For this review, take the finished solid that the model builds, in its own axes (mm). Face numbers are marked on the shaded views. A direction names the side the tool comes from. Round coordinates to 2 decimals unless told otherwise and drop trailing zeros. Order: outer loops, then holes, each group sorted by start corner. A loop starts at its lowest first (then second) coordinate and runs counter-clockwise, first axis right, second up. Notation, with made-up numbers: (10.5, 40) -> (42.5, 40) arc R28 ccw to (42.5, 64) -> close; hole circle Ø8 at (-17.75, 25). An arc over 180 degrees is marked (long way). Answer in a Markdown table with one row per item.
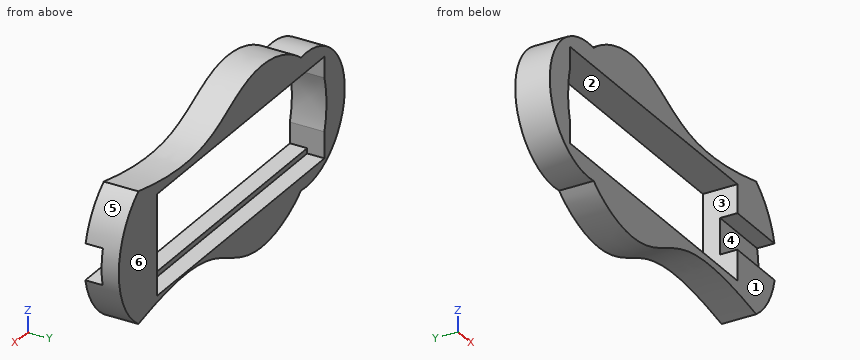
```python
from build123d import *

# Parameters (mm, degrees)
BOSS_EXTRUDE1_DEPTH = 20
SKETCH4_W           = 165
SKETCH4_H           = 3
CUT_EXTRUDE1_DEPTH  = 10
SKETCH9_W           = 41.41609898
SKETCH9_H           = 20.816936128
CUT_EXTRUDE2_DEPTH  = 10


with BuildPart() as part:
    # Sketch1 → Boss-Extrude1 (new body)
    with BuildSketch(Plane(origin=(0, 0, 0), x_dir=(1, 0, 0), z_dir=(0, 1, 0))):
        with BuildLine():
            add(Edge.make_bspline(
                [(145.295936906, 60.832177948), (44.156138469, 37.635123873), (68.598543861, 81.474917307), (14.861380224, 85.461006577), (-14.944677718, 60.924621218)],
                knots=[0, 0, 0, 0, 0, 1, 1, 1, 1, 1], degree=4))
            ThreePointArc((-14.944677718, 60.924621218), (-58.213287959, 23.039876711), (-14.944677718, -14.844867796))
            add(Edge.make_bspline(
                [(145.295936906, -14.752424526), (44.156138469, 8.444629549), (68.598543861, -35.395163885), (14.861380224, -39.381253155), (-14.944677718, -14.844867796)],
                knots=[0, 0, 0, 0, 0, 1, 1, 1, 1, 1], degree=4))
            ThreePointArc((145.295936906, -14.752424526), (164.569452441, 23.039876711), (145.295936906, 60.832177948))
        make_face()
        with BuildLine():
            Line((-38.21027036, -4.460123289), (-38.21027036, 7.689608728))
            add(Edge.make_bspline(
                [(-38.21027036, 38.390144694), (-42.352238314, 23.039876711), (-38.21027036, 7.689608728)],
                knots=[4.204471846, 4.204471846, 4.204471846, 5.220306115, 5.220306115, 5.220306115], degree=2, weights=[1, 0.873759421, 1]))
            Line((-38.21027036, 38.390144694), (-38.21027036, 50.539876711))
            Line((-38.21027036, 50.539876711), (126.78972964, 50.539876711))
            Line((126.78972964, 50.539876711), (126.78972964, -4.460123289))
            Line((126.78972964, -4.460123289), (-38.21027036, -4.460123289))
        make_face(mode=Mode.SUBTRACT)
    extrude(amount=BOSS_EXTRUDE1_DEPTH)

    # Sketch4 → Cut-Extrude1 (cut)
    with BuildSketch(Plane(origin=(0, 20, 0), x_dir=(1, 0, 0), z_dir=(0, 1, 0))):
        with Locations((44.28972964, 52.039876711)):
            Rectangle(SKETCH4_W, SKETCH4_H)
    extrude(amount=-CUT_EXTRUDE1_DEPTH, mode=Mode.SUBTRACT)

    # Sketch9 → Cut-Extrude2 (cut)
    with BuildSketch(Plane.XZ):
        with Locations((147.49777913, -22.403788733)):
            Rectangle(SKETCH9_W, SKETCH9_H)
    extrude(amount=-CUT_EXTRUDE2_DEPTH, mode=Mode.SUBTRACT)


solid = part.part
```
Q1. To check wall thickness, follow probe 1 along Z at (x, y) = (61, 1.5); probe 2 along X at (y, z) = (9.75, 2.5); probe 3 along Z at (x, y) = (24, 1). State the ranges of each line that lie inside material, in increasing order.
Answer key:
| item | result |
|---|---|
| probe 1 | z = -63.13 to -50.54, 4.46 to 17.05 |
| probe 2 | x = -48.43 to -38.21, 126.79 to 156.96 |
| probe 3 | z = -74.72 to -50.54, 4.46 to 28.64 |
Q2. Tool access review of the marked faces 1 and 2: name each direction out of +Z, -Z, +X, -X, +Y, -Y from which nothing blocks a thin tool from reaching the whole face with its end or side.
Answer key:
| item | result |
|---|---|
| face 1 | +Z, -Z, +X, -X, -Y |
| face 2 | +Y, -Y |
Q3. Take a section at B-B, the plane x = 149. Write out the cut boundary in (y, z), then the cut area to 3 significant figures.
Answer key:
| item | result |
|---|---|
| outline | (0, -57.85) -> (20, -57.85) -> (20, 11.77) -> (0, 11.77) -> (0, -12) -> (10, -12) -> (10, -32.81) -> (0, -32.81) -> close |
| area | 1,180 mm^2 |
Q4. Clearance check with flat-ended pins moving along their axes: pin 1 Ø11 at (x, y) = (146, 5) entering from +Z; pin 2 Ø6 at (x, z) = (144.5, -21) entering from -Y; pin 3 Ø5 at (x, y) = (4, 17) entering from +Z. State where each tip first meets the part, or that it passes through.
Answer key:
| item | result |
|---|---|
| pin 1 | stops at z = 14.75 |
| pin 2 | stops at y = 10 |
| pin 3 | stops at z = 26.11 |
Q5. Take a section at A-A, the plane z = -43.5. Write out the cut boundary in (x, y).
Answer key:
| item | result |
|---|---|
| outline | (-52.28, 0) -> (-38.21, 0) -> (-38.21, 20) -> (-52.28, 20) -> close; (126.79, 0) -> (159.85, 0) -> (159.85, 20) -> (126.79, 20) -> close |
Q6. The part is to be moulded in two halves that separate along Z. For the marked faces 3, 4, 5 and 6, say which applies: +Z half, -Z half, draft (parallel to the pull), parting line (faces both ways), or undercut.
Answer key:
| item | result |
|---|---|
| face 3 | undercut |
| face 4 | undercut |
| face 5 | parting line |
| face 6 | draft |
